from build123d import *

# Parameters (mm, degrees)
SKETCH1_W             = 100
SKETCH1_H             = 80
BOSS_EXTRUDE1_DEPTH   = 138
SKETCH2_W             = 100
SKETCH2_H             = 50
CUT_EXTRUDE1_DEPTH    = 8
M6_TAPPED_HOLE1_D     = 5
M6_TAPPED_HOLE1_DEPTH = 15
M6_TAPPED_HOLE1_TIP   = 1.502151548
SKETCH6_R             = 30
CUT_EXTRUDE2_DEPTH    = 168.164589552
M6_TAPPED_HOLE2_D     = 5
M6_TAPPED_HOLE2_DEPTH = 15
M6_TAPPED_HOLE2_TIP   = 1.502151548
M6_TAPPED_HOLE3_D     = 5
M6_TAPPED_HOLE3_DEPTH = 10
M6_TAPPED_HOLE3_TIP   = 1.502151548
M6_TAPPED_HOLE4_D     = 5
M6_TAPPED_HOLE4_DEPTH = 15
M6_TAPPED_HOLE4_TIP   = 1.502151548
CHAMFER1_SIZE         = 3


with BuildPart() as part:
    # Sketch1 → Boss-Extrude1 (new body)
    with BuildSketch(Plane(origin=(0, 0, 0), x_dir=(1, 0, 0), z_dir=(0, 1, 0))):
        Rectangle(SKETCH1_W, SKETCH1_H)
    extrude(amount=BOSS_EXTRUDE1_DEPTH)

    # Sketch2 → Cut-Extrude1 (cut)
    with BuildSketch(Plane.XZ):
        with Locations((0, -15)):
            Rectangle(SKETCH2_W, SKETCH2_H)
    extrude(amount=-CUT_EXTRUDE1_DEPTH, mode=Mode.SUBTRACT)

    # M6 Tapped Hole1
    with Locations(Plane(origin=(0, 8, 0), x_dir=(-1, 0, 0), z_dir=(0, -1, 0))):
        with Locations((-40, 25), (-40, 0), (40, 0), (40, 25)):
            Hole(M6_TAPPED_HOLE1_D / 2, depth=M6_TAPPED_HOLE1_DEPTH)
            with Locations((0, 0, -(M6_TAPPED_HOLE1_DEPTH + M6_TAPPED_HOLE1_TIP / 2))):  # 118° drill point
                Cone(0, M6_TAPPED_HOLE1_D / 2, M6_TAPPED_HOLE1_TIP, mode=Mode.SUBTRACT)

    # Sketch6 → Cut-Extrude2 (cut, through all)
    with BuildSketch(Plane(origin=(0, 0, -40), x_dir=(-1, 0, 0), z_dir=(0, 0, -1))):
        with Locations((0, 58)):
            Circle(SKETCH6_R)
    extrude(amount=-CUT_EXTRUDE2_DEPTH, mode=Mode.SUBTRACT)

    # M6 Tapped Hole2
    with Locations(Plane(origin=(0, 138, 0), x_dir=(1, 0, 0), z_dir=(0, 1, 0))):
        with Locations((-40, 30), (-40, -30), (40, -30), (40, 30)):
            Hole(M6_TAPPED_HOLE2_D / 2, depth=M6_TAPPED_HOLE2_DEPTH)
            with Locations((0, 0, -(M6_TAPPED_HOLE2_DEPTH + M6_TAPPED_HOLE2_TIP / 2))):  # 118° drill point
                Cone(0, M6_TAPPED_HOLE2_D / 2, M6_TAPPED_HOLE2_TIP, mode=Mode.SUBTRACT)

    # M6 Tapped Hole3
    with Locations(Plane(origin=(0, 0, -40), x_dir=(-1, 0, 0), z_dir=(0, 0, -1))):
        with Locations((-35, 23), (-35, 93), (35, 93), (35, 23)):
            Hole(M6_TAPPED_HOLE3_D / 2, depth=M6_TAPPED_HOLE3_DEPTH)
            with Locations((0, 0, -(M6_TAPPED_HOLE3_DEPTH + M6_TAPPED_HOLE3_TIP / 2))):  # 118° drill point
                Cone(0, M6_TAPPED_HOLE3_D / 2, M6_TAPPED_HOLE3_TIP, mode=Mode.SUBTRACT)

    # M6 Tapped Hole4
    with Locations(Plane.XY.offset(40)):
        with Locations((-35, 93), (35, 93), (35, 23), (-35, 23)):
            Hole(M6_TAPPED_HOLE4_D / 2, depth=M6_TAPPED_HOLE4_DEPTH)
            with Locations((0, 0, -(M6_TAPPED_HOLE4_DEPTH + M6_TAPPED_HOLE4_TIP / 2))):  # 118° drill point
                Cone(0, M6_TAPPED_HOLE4_D / 2, M6_TAPPED_HOLE4_TIP, mode=Mode.SUBTRACT)

    # Chamfer1
    chamfer1_edges = [part.edges().sort_by_distance(p)[0] for p in [
        (0, 0, 40),
        (-50, 73, -40),
        (50, 73, -40),
    ]]
    chamfer(chamfer1_edges, length=CHAMFER1_SIZE)


solid = part.part
CAD build for the part. Positions are in the model's coordinates, mm. A direction names the side the tool comes from. Coordinates: 2 decimals unless noted, no trailing zeros. Write each loop counter-clockwise with the first axis right and the second up, starting at its lowest first coordinate (ties: lowest second). Pieces come first, ordered by that corner, then holes. Notation, with made-up numbers: M 14,19.25 L 24,19.25 A13 cw 24,42.25 Z; hole C 52.5,66 d4. An arc over 180 degrees is marked long. Answer as a JSON object with one key per item and string values. Group by question number.
1) Tool access for faces 1 (the face through (41.34, 15.6, -27.11)), 2 (the face through (34.67, 95.48, -34.93)), 3 (the face through (-41.34, 130.4, -32.11)): list every direction of +Z, -Z, +X, -X, +Y, -Y with a clear straight run to the whole face (end or side of a thin tool).
2) Saw through at C-C (z = 8). Write the cut outline in (x, y), plus the area to 3 significant figures.
3) Pin check, flat tips, straight feed: pin 1 Ø3 at (x, z) = (-40, -30) entering from -Y; pin 2 Ø3 at (x, y) = (-35, 93) entering from -Z; pin 3 Ø4 at (x, y) = (-9.5, 2.5) entering from -Z. Stop position of each tip, or through.
4) Saw through at A-A (x = 0). Write the cut outline in (y, z), plus the area to 3 significant figures.
5) Mould opens along Z. For faces 4 (the face through (36.34, 25.11, -34.93)), 5 (the face through (34.77, 93.37, -28.76)), 6 (the face through (38.66, 130.4, -32.11)) say: +Z half, -Z half, draft (parallel to the pull), parting line (faces both ways), or undercut.
6) Wall check: line 1 (Z direction, x = -40, y = 129); line 2 (X direction, y = 93, z = 36); line 3 (Z direction, x = 40, y = 16.5). Give the ranges that are in metal, low to high. Write a range as from..to.
7) Saw through at B-B (y = 58). Write the cut outline in (x, z).
8) Saw through at D-D (y = 38). Write the cut outline in (x, z), plus the area to 3 significant figures.
Values follow:
{
 "1": {"face 1": "-Y", "face 2": "-Z", "face 3": "+Y"},
 "2": {"outline": "M -50,8 L 50,8 L 50,138 L -50,138 Z; hole C 0,58 d60", "area": "10,200 mm2"},
 "3": {"pin 1": "stops at y = 8", "pin 2": "stops at z = -29.4", "pin 3": "stops at z = 10"},
 "4": {"outline": "M 0,10 L 8,10 L 8,-40 L 28,-40 L 28,40 L 3,40 L 0,37 Z; M 88,-40 L 138,-40 L 138,40 L 88,40 Z", "area": "5,840 mm2"},
 "5": {"face 4": "draft", "face 5": "-Z half", "face 6": "undercut"},
 "6": {"line 1": "z = -40..-32.5, -27.5..27.5, 32.5..40", "line 2": "x = -50..-37.5, -32.5..32.5, 37.5..50", "line 3": "z = -40..-27.5, -22.5..-2.5, 2.5..40"},
 "7": {"outline": "M -50,-37 L -47,-40 L -30,-40 L -30,40 L -50,40 Z; M 30,-40 L 47,-40 L 50,-37 L 50,40 L 30,40 Z"},
 "8": {"outline": "M -50,-37 L -47,-40 L -22.36,-40 L -22.36,40 L -50,40 Z; M 22.36,-40 L 47,-40 L 50,-37 L 50,40 L 22.36,40 Z", "area": "4,410 mm2"}
}
